from build123d import *

# Parameters (mm, degrees)
ESBO_O1_R                = 1.75
RESSALTO_EXTRUS_O1_DEPTH = 3
ESBO_O2_W                = 10
ESBO_O2_H                = 30
RESSALTO_EXTRUS_O2_DEPTH = 3


with BuildPart() as part:
    # Esboço1 → Ressalto-extrusão1 (new body)
    with BuildSketch(Plane.XY):
        with BuildLine():
            ThreePointArc((-0.475822638, -3.719689882), (3.744330631, 0.206126489), (-0.88125, 3.644982639))
            ThreePointArc((-0.88125, 3.644982639), (-2.928276933, 2.342582807), (-3.749526707, 0.059577464))
            ThreePointArc((-3.749526707, 0.059577464), (-2.965124722, -2.295764662), (-0.88125, -3.644982639))
            Line((-0.88125, -3.644982639), (-0.496863485, -3.737916035))
            Line((-0.496863485, -3.737916035), (-0.475822638, -3.719689882))
        make_face()
        Circle(ESBO_O1_R, mode=Mode.SUBTRACT)
        with BuildLine():
            Line((8.5665, 5.929171759), (-0.88125, 3.644982639))
            ThreePointArc((-0.88125, 3.644982639), (3.744330631, 0.206126489), (-0.475822638, -3.719689882))
            Line((-0.475822638, -3.719689882), (-0.496863485, -3.737916035))
            Line((-0.496863485, -3.737916035), (8.5665, -5.929171759))
            ThreePointArc((8.5665, -5.929171759), (9.778798941, -6.095988032), (11, -6.017474553))
            Line((11, -6.017474553), (11, -3.97617907))
            ThreePointArc((11, -3.97617907), (5.9, 0), (11, 3.97617907))
            Line((11, 3.97617907), (11, 6.017474553))
            ThreePointArc((11, 6.017474553), (9.778798941, 6.095988032), (8.5665, 5.929171759))
        make_face()
        with BuildLine():
            ThreePointArc((-0.88125, -3.644982639), (-2.965124722, -2.295764662), (-3.749526707, 0.059577464))
            Line((-3.749526707, 0.059577464), (-17.354889152, -11.725757183))
            Line((-17.354889152, -11.725757183), (-14.081185083, -15.505024529))
            Line((-14.081185083, -15.505024529), (-0.496863485, -3.737916035))
            Line((-0.496863485, -3.737916035), (-0.88125, -3.644982639))
        make_face()
    extrude(amount=RESSALTO_EXTRUS_O1_DEPTH)

    # Esboço2 → Ressalto-extrusão2 (add)
    with BuildSketch(Plane(origin=(1.636852034, -1.889633673, 0), x_dir=(0.755853469, 0.654740814, 0), z_dir=(0.654740814, -0.755853469, 0))):
        with Locations((-15.795084972, 15)):
            Rectangle(ESBO_O2_W, ESBO_O2_H)
        with BuildLine():
            Line((-14.095084972, 26), (-14.095084972, 10))
            ThreePointArc((-14.095084972, 10), (-15.795084972, 8.3), (-17.495084972, 10))
            Line((-17.495084972, 10), (-17.495084972, 26))
            ThreePointArc((-17.495084972, 26), (-15.795084972, 27.7), (-14.095084972, 26))
        make_face(mode=Mode.SUBTRACT)
    extrude(amount=-RESSALTO_EXTRUS_O2_DEPTH)


solid = part.part
Here's how the part is built. I have some questions about the finished solid (model axes, mm). A direction names the side the tool comes from. Round coordinates to 2 decimals unless told otherwise and drop trailing zeros. Order: outer loops, then holes, each group sorted by start corner. A loop starts at its lowest first (then second) coordinate and runs counter-clockwise, first axis right, second up. Notation, with made-up numbers: M 81,20.25 L 87,20.25 A27 cw 87,37.25 Z; hole C 37,5 d10. An arc over 180 degrees is marked long. Return JSON: item names as keys, results as strings. Group by question number.
1. If we section it at B-B on x = 10: List the corners of the cut face in (y, z) for me.
2. On a 3-axis mill with a long thin cutter (end or side, diameter ignored), from which of +Z, -Z, +X, -X, +Y, -Y can I reach the whole of each face in a straight line? I mean faces 4 (the face through (-11.2, -11.1, 8.3)), 5 (the face through (3.971, -4.818, 1.479)), 6 (the face through (-7.49, -7.84, 16.31)), 7 (the face through (3.9, 4.8, 1.5)). Say none if no direction works.
3. If we section it at D-D on x = 4.5: List the corners of the cut face in (y, z) for me, then the cut area to 3 significant figures.
4. If we mould it in two halves opening along Z, with no side actions, what happens to faces 1 (the face through (-11.3, -11.1, 27.7)), 2 (the face through (-11, -11, 30)), 3 (the face through (1.617, -0.67, 1.479))? For each: pulls with the +Z half, pulls with the -Z half, needs draft (parallel to the pull), parting line crosses it, or undercut.
5. If we section it at A-A on z = 13.5: List the corners of the cut face in (x, y) for me.
6. Please list where these lines run through material, in increasing order: probe 1 along Y at (x, z) = (10, 2.35); probe 2 along Z at (x, y) = (-3.75, -2.5); probe 3 along Y at (x, z) = (-12.5, 27).
7. I'm going to push flat-ended pins straight in: pin 1 Ø6 at (x, y) = (-1.5, -5.5) entering from +Z; pin 2 Ø12 at (x, z) = (-6.5, 10.5) entering from +Y. Where does each tip first touch, or does it pass through?
8. If we section it at C-C on z = 5.5: List the corners of the cut face in (x, y) for me, then the cut area to 3 significant figures.
Reply:
{
 "1": {"outline": "M -6.1,0 L -4.1,0 L -4.1,3 L -6.1,3 Z; M 4.1,0 L 6.1,0 L 6.1,3 L 4.1,3 Z"},
 "2": {"face 4": "none", "face 5": "+Z, -Z, -Y", "face 6": "+Z, +X, +Y", "face 7": "+Z, -Z, -X, +Y"},
 "3": {"outline": "M -4.95,0 L 4.95,0 L 4.95,3 L -4.95,3 Z", "area": "29.7 mm^2"},
 "4": {"face 1": "undercut", "face 2": "pulls with the +Z half", "face 3": "needs draft"},
 "5": {"outline": "M -16.05,-13.24 L -14.08,-15.51 L -11.59,-13.34 L -13.55,-11.08 Z; M -10.98,-8.85 L -9.02,-11.12 L -6.52,-8.96 L -8.49,-6.69 Z"},
 "6": {"probe 1": "-6.1 to -4.1, 4.1 to 6.1", "probe 2": "0 to 3", "probe 3": "-14.14 to -11.79"},
 "7": {"pin 1": "z = 3", "pin 2": "y = -6.69"},
 "8": {"outline": "M -16.05,-13.24 L -14.08,-15.51 L -6.52,-8.96 L -8.49,-6.69 Z", "area": "30.0 mm^2"}
}
